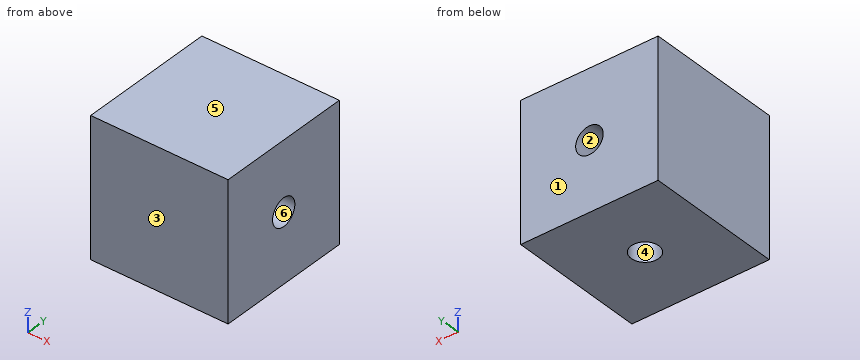
```python
from build123d import *

# Parameters (mm, degrees)
F0_W     = 15.24
F0_H     = 15.24
F1_DEPTH = 7.62
F3_D     = 3.048
F3_DEPTH = 10.16
F3_TIP   = 0.9157115834
F5_D     = 3.048
F5_DEPTH = 10.16
F5_TIP   = 0.9157115834
F7_D     = 3.048
F7_DEPTH = 10.16
F7_TIP   = 0.9157115834


with BuildPart() as f1:
    # F0 (on Front) → F1 (new body, symmetric)
    with BuildSketch(Plane.XZ):
        Rectangle(F0_W, F0_H)
    extrude(amount=F1_DEPTH, both=True)

    # F3 (one way)
    with BuildSketch(Plane.XY):
        with Locations((0, 0)):
            Circle(F3_D / 2)
    extrude(amount=-F3_DEPTH, mode=Mode.SUBTRACT)
    with Locations(Plane.XY):
        with Locations((0, 0)):
            with Locations((0, 0, -(F3_DEPTH + F3_TIP / 2))):  # 118° drill point
                Cone(0, F3_D / 2, F3_TIP, mode=Mode.SUBTRACT)

    # F5
    with Locations(Plane.YZ.offset(7.62)):
        with Locations((0, 0)):
            Hole(F5_D / 2, depth=F5_DEPTH)
            with Locations((0, 0, -(F5_DEPTH + F5_TIP / 2))):  # 118° drill point
                Cone(0, F5_D / 2, F5_TIP, mode=Mode.SUBTRACT)

    # F7
    with Locations(Plane(origin=(0, 7.62, 0), x_dir=(-1, 0, 0), z_dir=(0, 1, 0))):
        with Locations((0, 0)):
            Hole(F7_D / 2, depth=F7_DEPTH)
            with Locations((0, 0, -(F7_DEPTH + F7_TIP / 2))):  # 118° drill point
                Cone(0, F7_D / 2, F7_TIP, mode=Mode.SUBTRACT)


solid = f1.part
```
Model file for the job. Use its own axes, mm. Face numbers are marked on the shaded views. A direction names the side the tool comes from. Coordinates: 2 decimals unless noted, no trailing zeros. Order: outer loops, then holes, each group sorted by start corner. A loop starts at its lowest first (then second) coordinate and runs counter-clockwise, first axis right, second up. Notation, with made-up numbers: (20.25, 82) -> (26.25, 82) arc R31 ccw to (26.25, 118) -> close; hole circle Ø7 at (67, 44). An arc over 180 degrees is marked (long way). Return JSON: item names as keys, results as strings.
Item 1: Pin check, flat tip, straight feed: P1, Ø4, axis at x = 0, y = 0, coming from the -Z side. Stop position of the tip, or through.
Model answer:
{"P1": "stops at z = -7.62"}
Item 2: Mould opens along Y. For the marked faces 1, 2, 3 and 4 say: pulls with the +Y half, pulls with the -Y half, needs draft (parallel to the pull), parting line crosses it, or undercut.
Model answer:
{"face 1": "pulls with the +Y half", "face 2": "needs draft", "face 3": "pulls with the -Y half", "face 4": "undercut"}
Item 3: Wall check: line 1 along Y through (x, z) = (4, 0). Give the ranges that are in metal, low to high. Write a range as from..to.
Model answer:
{"line 1": "y = -7.62..-1.52, 1.52..7.62"}
Item 4: Slice it at A-A (y = 3.25). Write the cut outline in (x, z), then the cut area to 3 significant figures.
Model answer:
{"outline": "(-7.62, -7.62) -> (7.62, -7.62) -> (7.62, 7.62) -> (-7.62, 7.62) -> close; hole circle Ø3.05 at (0, 0)", "area": "225 mm²"}
Item 5: 3-axis set-ups, long thin cutter, end or side, ignore diameter. For the marked faces 5 and 6: which of +Z, -Z, +X, -X, +Y, -Y reach the whole face in a straight line?
Model answer:
{"face 5": "+Z, +X, -X, +Y, -Y", "face 6": "+X"}
